```python
from build123d import *

# Parameters (mm, degrees)
F2_R = 0.5


with BuildPart() as f1:
    # F0 (on Front) → F1 (revolve)
    with BuildSketch(Plane.XZ):
        Polygon((20.5, 5.5), (13.5, 5.5), (13.5, -5.5), (32.5, -5.5), (32.5, 0.5), (20.5, 0.5), align=None)
    revolve(axis=Axis((0, 0, -0.180863), (0, 0, -1)))

    # F2
    f2_edges = [f1.edges().sort_by_distance(p)[0] for p in [
        (-32.5, 0, -5.5),
        (-32.5, 0, 0.5),
        (-20.5, 0, 5.5),
        (-20.5, 0, 0.5),
    ]]
    fillet(f2_edges, radius=F2_R)


solid = f1.part
```
CAD build for the part. Positions are in the model's coordinates, mm. A direction names the side the tool comes from. Coordinates: 2 decimals unless noted, no trailing zeros. Write each loop counter-clockwise with the first axis right and the second up, starting at its lowest first coordinate (ties: lowest second). Pieces come first, ordered by that corner, then holes.
(1) 3-axis set-ups, long thin cutter, end or side, ignore diameter. For faces 4 (the face through (-4.444, 20.013, 3.028)), 5 (the face through (13.1, 4.2, 5.5)): which of +Z, -Z, +X, -X, +Y, -Y reach the whole face in a straight line?
(2) Cut at C-C, the plane z = 2.25. List the corners of the cut face in (x, y).
(3) Flat gauge pins, fed straight in: pin 1 (1 mm diameter, centred on x = -6, z = -4, fed in from -Y); pin 2 (4 mm diameter, centred on y = 22.5, z = -3, fed in from +X); pin 3 (1 mm diameter, centred on y = 22.5, z = 2, fed in from +X); pin 4 (4 mm diameter, centred on y = -19.5, z = 1, fed in from -X). Where does each tip first touch, or does it go through?
(4) Drill centre lines: probe 1 along Y at (x, z) = (0, -2); probe 2 along X at (y, z) = (0, 1.5). Where is each one in solid material? Low to high.
(5) Two-plate mould, pull along Y, no slides. Class faces 1 (the face through (21, 7, 0.5)), 2 (the face through (31, -9.76, -2.46)), 3 (the face through (-2.93, 13.18, -0.08)): +Y half, -Y half, draft (parallel to the pull), parting line (faces both ways), or undercut.
(6) Cut at D-D, the plane z = -2.25. List the corners of the cut face in (x, y).
(7) Cut at A-A, the plane y = 0. List the corners of the cut face in (x, z), and give its area (3 significant figures).
Geometry says:
1. face 4: +Z
1. face 5: +Z, +X, -X, +Y, -Y
2. outline: circle Ø41 at (0, 0); hole circle Ø27 at (0, 0)
3. pin 1: stops at y = -32.03
3. pin 2: stops at x = 25.22
3. pin 3: passes through
3. pin 4: stops at x = -27.24
4. probe 1: y = -32.5 to -13.5, 13.5 to 32.5
4. probe 2: x = -20.5 to -13.5, 13.5 to 20.5
5. face 1: draft
5. face 2: parting line
5. face 3: undercut
6. outline: circle Ø65 at (0, 0); hole circle Ø27 at (0, 0)
7. outline: (-32.5, -5) arc R0.5 ccw to (-32, -5.5) - (-13.5, -5.5) - (-13.5, 5.5) - (-20, 5.5) arc R0.5 ccw to (-20.5, 5) - (-20.5, 1) arc R0.5 cw to (-21, 0.5) - (-32, 0.5) arc R0.5 ccw to (-32.5, 0) - close; (13.5, -5.5) - (32, -5.5) arc R0.5 ccw to (32.5, -5) - (32.5, 0) arc R0.5 ccw to (32, 0.5) - (21, 0.5) arc R0.5 cw to (20.5, 1) - (20.5, 5) arc R0.5 ccw to (20, 5.5) - (13.5, 5.5) - close
7. area: 298 mm2
